Check sheet for the modelled part. Datum: model origin and axes. Units: mm. Give positions to 0.01 mm unless a question says otherwise; leave off trailing zeros. Write each loop counter-clockwise with the first axis right and the second up, starting at its lowest first coordinate (ties: lowest second). Pieces come first, ordered by that corner, then holes.
Autodesk Fusion 360 part; units mm, degrees
sketch "スケッチ1" plane through (0, 0, 0) normal (0, 0, 1) x (1, 0, 0)
  line L0 (0, 0) -> (72.5, 0)
  line L1 (0, 0) -> (0, 35)
  line L2 (0, 35) -> (30, 35)
  line L3 (30, 35) -> (72.5, 0)
  line L4 (72.5, 0) -> (74.0893, 1.9298)
  line L5 (74.0893, 1.9298) -> (31.5893, 36.9298)
  line L6 (31.5893, 36.9298) -> (30, 35)
  line L7 (31.5893, 36.9298) -> (0, 36.9298)
  line L8 (31.5893, 36.9298) -> (-4, 42)
  line L9 (31.5893, 36.9298) -> (74.0893, 1.9298)
  line L10 (31.5893, 36.9298) -> (90.0627, 19.4298)
  line L11 (0, 0) -> (0, -10)
  line L12 (0, -10) -> (105, -10)
  line L13 (74.0893, 1.9298) -> (88.5755, -10)
  line L14 (72.5, 0) -> (84.6429, -10)
  dimension "d1" = 72.5
  dimension "d2" = 35
  dimension "d3" = 30
  dimension "d4" = 2.5
  dimension "d5" = 10
revolve "回転1" add sketch "スケッチ1" angle 359.9 about axis through (0, 0, 0) along (0, 1, 0) contours L3 L4 L5 L6 L9
extrude "押し出し1" add 1 faces at (45.2261, 24.6199, 0.0789) along direction (0.001745, 0, 0.999998) blind 0.05
1) Scan lines: L1, parallel to Z at x = -15.5, y = 24; L2, parallel to Z at x = -12.5, y = 18; L3, parallel to X at y = 4, z = 26. Record each from-to range of solid material in increasing order.
2) Sectioned sample at B-B on y = 8. Record the boundary of the cut face in (x, z), then the cut area to 3 significant figures.
3) Gauge pin test, flat ends, axial feed: pin 1 (5 mm diameter, centred on x = -44, y = 15.5, fed in from -Z); pin 2 (8 mm diameter, centred on x = -31.5, z = 50.5, fed in from -Y); pin 3 (4 mm diameter, centred on x = 32, y = 24, fed in from -Z). Record the tip position at first contact, or that the pin passes through.
4) Sectioned sample at A-A on x = 0. Record the boundary of the cut face in (y, z).
5) Sectioned sample at C-C on y = 27.5. Record the boundary of the cut face in (x, z), then the cut area to 3 significant figures.
Answers below:
1. L1: z = -44.68 to -40.49, 40.49 to 44.68
1. L2: z = -53.12 to -49.08, 49.08 to 53.12
1. L3: x = -66.69 to -62.45, 62.45 to 66.69
2. outline: (62.79, 0) arc R62.79 cw (long way) to (62.79, 0.16) - (62.79, 0.11) - (66.72, 0.12) arc R66.72 ccw (long way) to (66.72, 0) - close
2. area: 1,600 mm2
3. pin 1: stops at z = -42.44
3. pin 2: stops at y = 7.4
3. pin 3: stops at z = -38.46
4. outline: (0, -72.5) - (1.93, -74.09) - (36.93, -31.59) - (35, -30) - close; (0, 72.5) - (35, 30) - (36.93, 31.59) - (1.93, 74.09) - close
5. outline: (39.11, 0) arc R39.11 cw (long way) to (39.11, 0.12) - (39.11, 0.07) - (43.04, 0.08) arc R43.04 ccw (long way) to (43.04, 0) - close
5. area: 1,010 mm2
